The listing builds one solid part. Answer for the finished solid, in the listing's coordinates (mm). A direction names the side the tool comes from. Coordinates: 2 decimals unless noted, no trailing zeros. Write each loop counter-clockwise with the first axis right and the second up, starting at its lowest first coordinate (ties: lowest second). Pieces come first, ordered by that corner, then holes.
from build123d import *

# Parameters (mm, degrees)
F1_DEPTH = 57.15
F2_R     = 5.715
F3_DEPTH = 5.08
F4_R     = 6.985
F5_DEPTH = 2.54
F7_DEPTH = 5.08


with BuildPart() as f1:
    # F0 (on Right) → F1 (new body)
    with BuildSketch(Plane.YZ):
        with BuildLine():
            Line((0, 10.16), (0, 1.27))
            ThreePointArc((0, 1.27), (0.371974, 0.371974), (1.27, 0))
            Line((1.27, 0), (1.905, 0))
            ThreePointArc((1.905, 0), (2.803026, 0.371974), (3.175, 1.27))
            Line((3.175, 1.27), (3.175, 9.525))
            ThreePointArc((3.175, 9.525), (3.972931, 11.858139), (6.0325, 13.214017))
            ThreePointArc((6.0325, 13.214017), (6.719023, 13.665976), (6.985, 14.443689))
            Line((6.985, 14.443689), (6.985, 15.24))
            ThreePointArc((6.985, 15.24), (6.613026, 16.138026), (5.715, 16.51))
            Line((5.715, 16.51), (1.27, 16.51))
            ThreePointArc((1.27, 16.51), (0.371974, 16.138026), (0, 15.24))
            Line((0, 15.24), (0, 10.16))
        make_face()
    extrude(amount=F1_DEPTH)

    # F2 (on face) → F3 (join)
    with BuildSketch(Plane.XZ):
        with BuildLine():
            ThreePointArc((28.575, 1.27), (33.514141, 3.315859), (35.56, 8.255))
            ThreePointArc((35.56, 8.255), (33.514141, 13.194141), (28.575, 15.24))
            ThreePointArc((28.575, 15.24), (21.59, 8.255), (28.575, 1.27))
        make_face()
        with Locations((28.575, 8.255)):
            Circle(F2_R, mode=Mode.SUBTRACT)
    extrude(amount=F3_DEPTH)

    # F4 (on face) → F5 (join)
    with BuildSketch(Plane.XZ.offset(5.08)):
        with Locations((28.575, 8.255)):
            Circle(F4_R)
    extrude(amount=F5_DEPTH)

    # F6 (on face) → F7 (cut)
    with BuildSketch(Plane.XZ.offset(7.62)):
        with BuildLine():
            Line((30.48, 13.335), (28.575, 13.335))
            Line((28.575, 13.335), (26.67, 13.335))
            ThreePointArc((26.67, 13.335), (24.873949, 12.591051), (24.13, 10.795))
            Line((24.13, 10.795), (24.13, 5.715))
            ThreePointArc((24.13, 5.715), (24.873949, 3.918949), (26.67, 3.175))
            Line((26.67, 3.175), (30.48, 3.175))
            ThreePointArc((30.48, 3.175), (32.276051, 3.918949), (33.02, 5.715))
            Line((33.02, 5.715), (33.02, 8.255))
            Line((33.02, 8.255), (33.02, 10.795))
            ThreePointArc((33.02, 10.795), (32.276051, 12.591051), (30.48, 13.335))
        make_face()
    extrude(amount=-F7_DEPTH, mode=Mode.SUBTRACT)


solid = f1.part
Q1. Which of the six approach directions +Z, -Z, +X, -X, +Y, -Y give full straight-line access (tool end or side, diameter ignored) to faces 4 (the face through (27.83, -2.5, 13.92)), 5 (the face through (28.17, 6.62, 16.13)), 6 (the face through (33.02, -6, 8))?
Answers below:
face 4: none
face 5: +Z, +X, -X, +Y
face 6: -Y
Q2. Given pin 1 (6.5 mm diameter, centred on x = 29.5, z = 7, fed in from +Y); pin 2 (7 mm diameter, centred on x = 40.5, z = 6.5, fed in from -Y); pin 3 (1.3 mm diameter, centred on x = 28, y = -6.5, fed in from +Z), each flat-ended and moving along its own axis, determine where each tip first touches the part or whether it passes through.
Answers below:
pin 1: stops at y = 3.24
pin 2: stops at y = 0
pin 3: stops at z = 15.24
Q3. The part is cut by section B-B, the plane y = -5.75. Write down the section's boundary in (x, z) (3 decimals).
Answers below:
outline: circle Ø13.97 at (28.575, 8.255); hole (24.13, 5.715) arc R2.54 ccw to (26.67, 3.175) - (30.48, 3.175) arc R2.54 ccw to (33.02, 5.715) - (33.02, 10.795) arc R2.54 ccw to (30.48, 13.335) - (26.67, 13.335) arc R2.54 ccw to (24.13, 10.795) - close
Q4. Find the intervals of material crossed by probe 1 along Y at (x, z) = (30, 4.5) (3 decimals); probe 2 along Y at (x, z) = (34.5, 5.25) (3 decimals); probe 3 along Z at (x, y) = (31, -6.5), in increasing order.
Answers below:
probe 1: y = 0 to 3.175
probe 2: y = -7.62 to 3.175
probe 3: z = 1.7 to 3.23, 13.28 to 14.81
Q5. Determine the mould class of faces 1 (the face through (28, 3.175, 5)), 2 (the face through (29, -6, 13.335)), 3 (the face through (57.15, 3, 10)) for opening direction X: released by +X, released by -X, zero draft, split by the parting line, or undercut.
Answers below:
face 1: zero draft
face 2: undercut
face 3: released by +X
Q6. The part is cut by section A-A, the plane x = 10. Write down the section's boundary in (y, z) (1 decimal).
Answers below:
outline: (0, 1.3) arc R1.3 ccw to (1.3, 0) - (1.9, 0) arc R1.3 ccw to (3.2, 1.3) - (3.2, 9.5) arc R3.8 cw to (6, 13.2) arc R1.3 ccw to (7, 14.4) - (7, 15.2) arc R1.3 ccw to (5.7, 16.5) - (1.3, 16.5) arc R1.3 ccw to (0, 15.2) - close
Q7. The part is cut by section D-D, the plane y = -1.5. Write down the section's boundary in (x, z) (3 decimals), then the cut area to 3 significant figures.
Answers below:
outline: circle Ø13.97 at (28.575, 8.255); hole circle Ø11.43 at (28.575, 8.255)
area: 50.7 mm2
